```python
from build123d import *

# Parameters (mm, degrees)
BOSS_EXTRUDE1_DEPTH = 54
FILLET1_R           = 20
FILLET2_R           = 5
SHELL1_T            = -4
BOSS_EXTRUDE2_REACH = 156.081
SKETCH2_W           = 29
SKETCH2_H           = 24
SKETCH3_W           = 19
SKETCH3_H           = 19
CUT_EXTRUDE1_DEPTH  = 54
FILLET3_R           = 3


with BuildPart() as part:
    # Sketch1 → Boss-Extrude1 (new body)
    with BuildSketch(Plane(origin=(0, 0, 0), x_dir=(0, 0, -1), z_dir=(1, 0, 0))):
        Polygon((0, 0), (29.368487091, 35), (140, 35), (140, 0), align=None)
    extrude(amount=BOSS_EXTRUDE1_DEPTH)

    # Fillet1
    fillet1_edges = [part.edges().sort_by_distance(p)[0] for p in [
        (27, 35, -29.368487091),
        (27, 35, -140),
    ]]
    fillet(fillet1_edges, radius=FILLET1_R)

    # Fillet2
    fillet2_edges = [part.edges().sort_by_distance(p)[0] for p in [
        (0, 35, -79.347320127),
        (54, 35, -79.347320127),
        (0, 13.927876097, -11.686875696),
        (0, 33.126155741, -30.242275019),
        (0, 29.142135624, -134.142135624),
        (54, 13.927876097, -11.686875696),
        (54, 33.126155741, -30.242275019),
        (54, 29.142135624, -134.142135624),
        (0, 7.5, -140),
        (54, 7.5, -140),
    ]]
    fillet(fillet2_edges, radius=FILLET2_R)

    # Shell1
    shell1_openings = [part.faces().sort_by_distance(p)[0] for p in [
        (27, 0, -70.029322897),
    ]]
    offset(amount=SHELL1_T, openings=shell1_openings, kind=Kind.INTERSECTION)

    # Boss-Extrude2: up to this face of the body (flat: up to its plane)
    boss_extrude2_end = Plane(part.part.faces().sort_by_distance((27, 13.927876097, -11.686875696))[0])
    # Sketch2 → Boss-Extrude2 (add, up to the picked face)
    with BuildSketch(Plane.XY, mode=Mode.PRIVATE) as boss_extrude2_sk1:
        with Locations((27, 12)):
            Rectangle(SKETCH2_W, SKETCH2_H)
    boss_extrude2_tool1 = split(extrude(boss_extrude2_sk1.sketch, amount=-BOSS_EXTRUDE2_REACH, mode=Mode.PRIVATE), bisect_by=boss_extrude2_end, keep=Keep.BOTH, mode=Mode.PRIVATE)
    add(boss_extrude2_tool1.solids().sort_by(Axis((27, 12, 0), (0, 0, -1)))[0])

    # Sketch3 → Cut-Extrude1 (cut)
    with BuildSketch(Plane.XY):
        with Locations((27, 9.5)):
            Rectangle(SKETCH3_W, SKETCH3_H)
    extrude(amount=-CUT_EXTRUDE1_DEPTH, mode=Mode.SUBTRACT)

    # Fillet3
    fillet3_edges = [part.edges().sort_by_distance(p)[0] for p in [
        (41.5, 24, -10.069195574),
        (12.5, 24, -10.069195574),
    ]]
    fillet(fillet3_edges, radius=FILLET3_R)


solid = part.part
```
Geometry: final body of the model. Coordinates: model frame, mm. A direction names the side the tool comes from. Coordinates: 2 decimals unless noted, no trailing zeros. Loops run counter-clockwise (first coordinate to the right, second up) from the corner with the lowest first, then second, coordinate; pieces in that order, holes last. Notation, with made-up numbers: (46.25, 74.25) -> (60.25, 74.25) arc R8 cw to (60.25, 82.25) -> close; hole circle Ø10 at (-24, 58). An arc over 180 degrees is marked (long way). Use a Markdown table: item, result. Add a question column.
(1) Mould query, pull axis Z, two halves, no side actions, for faces 1 (the cylindrical face through (40.64, 23.1, -10.21)), 2 (the flat face through (4, 15, -72)), 3 (the cylindrical face through (27.308, 29.297, -133.986)). Classes: pulls with the +Z half, pulls with the -Z half, needs draft (parallel to the pull), parting line crosses it, or undercut.
(2) Pin query (flat end, axial travel): pin 1 Ø8 at (x, y) = (7, 16) entering from -Z; pin 2 Ø22 at (x, z) = (29, -62.5) entering from -Y; pin 3 Ø4.5 at (x, y) = (25, 8) entering from +Z; pin 4 Ø10 at (x, z) = (26.5, -7) entering from +Y. Return the tip coordinate at first contact, or that it passes through.
(3) Section query A-A, the plane x = 11. Return loops of the section in (y, z).
(4) Line query: line 1 along X through (y, z) = (30, -122); line 2 along X through (y, z) = (18.5, -15); line 3 along Y through (x, z) = (8.5, -54). Output: solid intervals per line, ascending.
(5) Access query for faces 4 (the cylindrical face through (4.285, 12.626, -16.209)), 5 (the cylindrical face through (13.4, 23.14, -10.21)), 6 (the flat face through (41.5, 15, -5)). Directions: +Z, -Z, +X, -X, +Y, -Y. A direction counts if a zero-diameter tool reaches every point of the face in a straight line with its end or side. Return the directions, or none.
(6) Section query C-C, the plane x = 33.5. Return loops of the section in (y, z).
(7) Section query B-B, the plane z = -71.5. Return loops of the section in (x, y), plus the area to 3 significant figures.
Answer:
| question | item | result |
|---|---|---|
| 1 | face 1 | needs draft |
| 1 | face 2 | undercut |
| 1 | face 3 | pulls with the -Z half |
| 2 | pin 1 | stops at z = -140 |
| 2 | pin 2 | stops at y = 31 |
| 2 | pin 3 | stops at z = -136 |
| 2 | pin 4 | stops at y = 24 |
| 3 | outline | (0, -140) -> (15, -140) arc R20 ccw to (35, -120) -> (35, -38.69) arc R20 ccw to (27.86, -23.37) -> (0, 0) -> (0, -5.22) -> (25.28, -26.44) arc R16 cw to (31, -38.69) -> (31, -120) arc R16 cw to (15, -136) -> (0, -136) -> close |
| 4 | line 1 | x = 0 to 4.01, 49.99 to 54 |
| 4 | line 2 | x = 12.5 to 17.5, 36.5 to 41.5 |
| 4 | line 3 | y = 31 to 35 |
| 5 | face 4 | -Y |
| 5 | face 5 | +Z, -X, +Y |
| 5 | face 6 | +Z, +X, +Y |
| 6 | outline | (0, -140) -> (15, -140) arc R20 ccw to (35, -120) -> (35, -38.69) arc R20 ccw to (27.86, -23.37) -> (24, -20.14) -> (24, 0) -> (19, 0) -> (19, -21.16) -> (25.28, -26.44) arc R16 cw to (31, -38.69) -> (31, -120) arc R16 cw to (15, -136) -> (0, -136) -> close |
| 7 | outline | (0, 0) -> (4, 0) -> (4, 30) arc R1 cw to (5, 31) -> (49, 31) arc R1 cw to (50, 30) -> (50, 0) -> (54, 0) -> (54, 30) arc R5 ccw to (49, 35) -> (5, 35) arc R5 ccw to (0, 30) -> close |
| 7 | area | 454 mm^2 |
